```python
from build123d import *

# Parameters (mm, degrees)
F1_DEPTH = 76.2


with BuildPart() as f1:
    # F0 (on Top) → F1 (new body)
    with BuildSketch(Plane.XY):
        with BuildLine():
            Line((0, 123.950441), (0, 1.5875))
            ThreePointArc((0, 1.5875), (0.464968, 0.464968), (1.5875, 0))
            Line((1.5875, 0), (181.374797, 0))
            Line((181.374797, 0), (194.302927, 0))
            ThreePointArc((194.302927, 0), (195.425459, 0.464968), (195.890427, 1.5875))
            Line((195.890427, 1.5875), (195.890427, 17.4625))
            ThreePointArc((195.890427, 17.4625), (195.425459, 18.585032), (194.302927, 19.05))
            ThreePointArc((194.302927, 19.05), (193.180395, 18.585032), (192.715427, 17.4625))
            Line((192.715427, 17.4625), (192.715427, 4.7625))
            ThreePointArc((192.715427, 4.7625), (192.250459, 3.639968), (191.127927, 3.175))
            Line((191.127927, 3.175), (176.840427, 3.175))
            Line((176.840427, 3.175), (2.498053, 125.250845))
            ThreePointArc((2.498053, 125.250845), (0.854474, 125.358571), (0, 123.950441))
        make_face()
        with BuildLine():
            Line((5.673053, 119.151726), (167.180629, 6.062904))
            ThreePointArc((167.180629, 6.062904), (167.784102, 4.28513), (166.270077, 3.175))
            Line((166.270077, 3.175), (4.7625, 3.175))
            ThreePointArc((4.7625, 3.175), (3.639968, 3.639968), (3.175, 4.7625))
            Line((3.175, 4.7625), (3.175, 117.851323))
            ThreePointArc((3.175, 117.851323), (4.029474, 119.259452), (5.673053, 119.151726))
        make_face(mode=Mode.SUBTRACT)
    extrude(amount=F1_DEPTH)


solid = f1.part
```
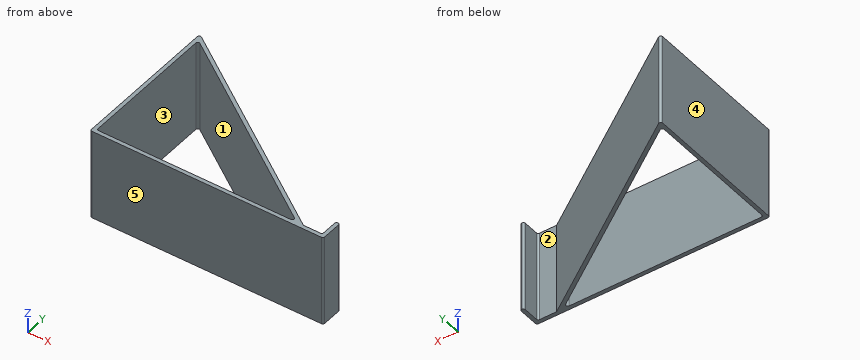
For this review, take the finished solid that the model builds, in its own axes (mm). Face numbers are marked on the shaded views. A direction names the side the tool comes from. Round coordinates to 2 decimals unless told otherwise and drop trailing zeros. Write each loop counter-clockwise with the first axis right and the second up, starting at its lowest first coordinate (ties: lowest second). Pieces come first, ordered by that corner, then holes. Notation, with made-up numbers: M 23,19.5 L 53,19.5 A34 cw 53,52.5 Z; hole C 13,30.5 d7. An arc over 180 degrees is marked long. One line per item, written item: value. Start each with the question number.
(1) Insertion check: pin 1 (10 mm diameter, centred on y = 57, z = 16, fed in from +X); pin 2 (1.5 mm diameter, centred on x = 53.5, z = 30.5, fed in from +Y); pin 3 (4.5 mm diameter, centred on x = 181, z = 39.5, fed in from +Y) (3 decimals). Each pin has a flat end and moves straight along its axis. Give the tip position at first contact, or say it passes through.
(2) Machinability: for the marked faces 1 and 2, which of the approach directions +Z, -Z, +X, -X, +Y, -Y give a long, thin tool a straight path to every point of the face, cutting with its end or side? Answer none if there is none.
(3) We need section B-B (y = 74). Give the boundary of the cut face in (x, z) (3 decimals).
(4) We need section C-C (x = 101). Give the boundary of the cut face in (y, z) (3 decimals), and give its area (3 significant figures).
(5) The part is to be moulded in two halves that separate along X. For the marked faces 3, 4 and 5, say which applies: released by +X, released by -X, zero draft, split by the parting line, or undercut.
(6) Wall thickness on line 1 (Y direction, x = 126, z = 16) (3 decimals); line 2 (Y direction, x = 160, z = 37.5) (3 decimals); line 3 (X direction, y = 78.5, z = 45) (3 decimals): over which ranges is each line inside the solid? List them lowest first.
Result:
1. pin 1: x = 107.11
1. pin 2: y = 90.06
1. pin 3: y = 3.175
2. face 1: +Z, -Z
2. face 2: +Z, -Z, +Y
3. outline: M 0,0 L 3.175,0 L 3.175,76.2 L 0,76.2 Z; M 70.156,0 L 75.692,0 L 75.692,76.2 L 70.156,76.2 Z
4. outline: M 0,0 L 3.175,0 L 3.175,76.2 L 0,76.2 Z; M 52.403,0 L 56.279,0 L 56.279,76.2 L 52.403,76.2 Z
4. area: 537 mm²
5. face 3: undercut
5. face 4: released by -X
5. face 5: zero draft
6. line 1: 0 to 3.175, 34.898 to 38.774
6. line 2: 0 to 3.175, 11.091 to 14.967
6. line 3: 0 to 3.175, 63.73 to 69.265
